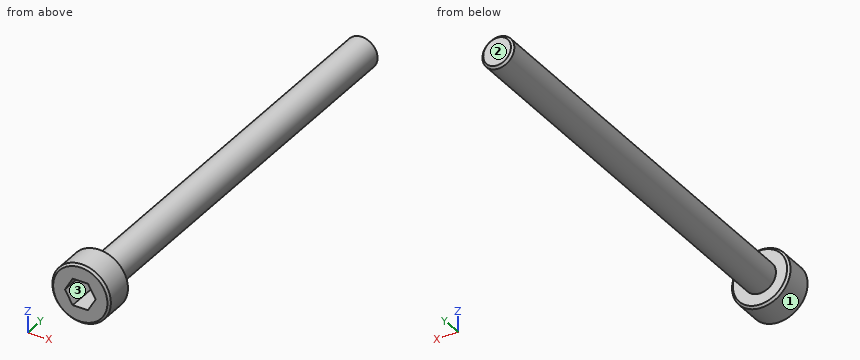
```python
from build123d import *

# Parameters (mm, degrees)
SKETCH006_R             = 2.75
PAD002_DEPTH            = 3
SKETCH007_R             = 1.5
PAD003_DEPTH            = 40
POCKET003_DEPTH         = 4
CHAMFER001_SIZE         = 0.2
BODY002_PLACEMENT_ANGLE = 90


with BuildPart() as part:
    # Sketch006 → Pad002 (new body)
    with BuildSketch(Plane.XY):
        Circle(SKETCH006_R)
    extrude(amount=PAD002_DEPTH)

    # Sketch007 (on Face2 of Pad002) → Pad003 (join)
    with BuildSketch(Plane(origin=(0, 0, 0), x_dir=(1, 0, 0), z_dir=(0, 0, -1))):
        Circle(SKETCH007_R)
    extrude(amount=PAD003_DEPTH)

    # Sketch008 (on DatumPlane) → Pocket003 (cut)
    with BuildSketch(Plane.XY.offset(3)):
        Polygon((0.7216878365, -1.25), (1.443375673, 0), (0.7216878365, 1.25), (-0.7216878365, 1.25), (-1.443375673, 0), (-0.7216878365, -1.25), align=None)
    extrude(amount=-POCKET003_DEPTH, mode=Mode.SUBTRACT)

    # Chamfer001
    chamfer001_edges = [part.edges().sort_by_distance(p)[0] for p in [
        (-1.5, 0, -40),
        (-2.75, 0, 0),
        (-2.75, 0, 3),
    ]]
    chamfer(chamfer001_edges, length=CHAMFER001_SIZE)


with BuildPart() as part_1:
    # Body002 placement: moved
    add(part.part.moved(Location((35.8, 0, 78.7))).rotate(Axis((35.8, 0, 78.7), (1, 0, 0)), BODY002_PLACEMENT_ANGLE))


solid = part_1.part
```
Work out the finished part from the listing and answer in its coordinate system (mm). Face numbers are marked on the shaded views. Coordinates: 2 decimals unless noted, no trailing zeros. Loops run counter-clockwise (first coordinate to the right, second up) from the corner with the lowest first, then second, coordinate; pieces in that order, holes last. Notation, with made-up numbers: (-14, -20.75) - (6, -20.75) arc R12 cw to (6, 1.25) - close; hole circle Ø10 at (86, 44). An arc over 180 degrees is marked (long way). Use a Markdown table: item, result.
Item 1: The mould has two halves that part along Z. Classify the marked faces 1, 2 and 3: +Z half, -Z half, draft (parallel to the pull), parting line (faces both ways), or undercut.
Evaluation:
| item | result |
|---|---|
| face 1 | parting line |
| face 2 | draft |
| face 3 | undercut |
Item 2: Find section B-B, the plane y = 10. Determine the outline of the cut face in (x, z), and give its area (3 significant figures).
Evaluation:
| item | result |
|---|---|
| outline | circle Ø3 at (35.8, 78.7) |
| area | 7.07 mm2 |
Item 3: Given pin 1 Ø0.8 at (x, z) = (36, 78.5) entering from -Y; pin 2 Ø1.5 at (y, z) = (7, 79.5) entering from -X; pin 3 Ø3 at (x, y) = (36, 18.5) entering from +Z, each flat-ended and moving along its own axis, determine where each tip first touches the part or whether it passes through.
Evaluation:
| item | result |
|---|---|
| pin 1 | stops at y = 1 |
| pin 2 | stops at x = 34.3 |
| pin 3 | stops at z = 80.2 |
Item 4: Find section A-A, the plane x = 35.8. Determine the outline of the cut face in (y, z), and give its area (3 significant figures).
Evaluation:
| item | result |
|---|---|
| outline | (-3, 76.15) - (-2.8, 75.95) - (-0.2, 75.95) - (0, 76.15) - (0, 77.2) - (39.8, 77.2) - (40, 77.4) - (40, 80) - (39.8, 80.2) - (0, 80.2) - (0, 81.25) - (-0.2, 81.45) - (-2.8, 81.45) - (-3, 81.25) - (-3, 79.95) - (1, 79.95) - (1, 77.45) - (-3, 77.45) - close |
| area | 126 mm2 |
Item 5: Consider probe 1 along Y at (x, z) = (36.7, 80.45); probe 2 along Z at (x, y) = (35.75, 7.5); probe 3 along Y at (x, z) = (36.4, 78.2). Determine where each line is inside the solid, lowest interval first. Write a range as from..to.
Evaluation:
| item | result |
|---|---|
| probe 1 | y = -3..0 |
| probe 2 | z = 77.2..80.2 |
| probe 3 | y = 1..40 |
